Verification items for this drawing (mm, ordinates from the low corner). Give positions to 0.01 mm unless a question says otherwise; leave off trailing zeros. Loops run counter-clockwise (first coordinate to the right, second up) from the corner with the lowest first, then second, coordinate; pieces in that order, holes last. Notation, with made-up numbers: M -6,27.5 L 49,27.5 A21 cw 49,66.5 Z; hole C -31.75,12 d6. An arc over 180 degrees is marked long. Use a Markdown table: item, result.
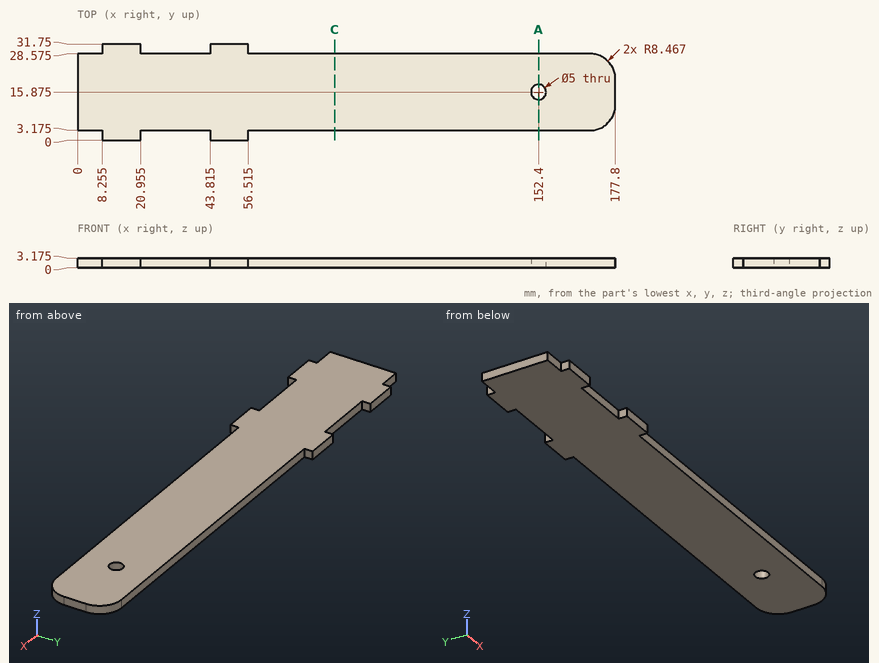
(1) Gauge pin test, flat ends, axial feed: P1, Ø1.6, axis at y = 30, z = 1, coming from the -X side (3 decimals); P2, Ø1, axis at x = 2.5, z = 2, coming from the -Y side (3 decimals); P3, Ø1.6, axis at x = 36.5, z = 1.5, coming from the +Y side (3 decimals). Record the tip position at first contact, or that the pin passes through.
Results below:
| item | result |
|---|---|
| P1 | x = 8.255 |
| P2 | y = 3.175 |
| P3 | y = 28.575 |
(2) Cross-section at C-C on x = 85. Record the cut outline in (y, z) (1 decimal).
Results below:
| item | result |
|---|---|
| outline | M 3.2,0 L 28.6,0 L 28.6,3.2 L 3.2,3.2 Z |
(3) Material ranges on line 1 (X direction, y = 16, z = 2.2); line 2 (Y direction, x = 152.4, z = 1.3) (1 decimal); line 3 (X direction, y = 2, z = 2.35) (1 decimal), recorded low to high.
Results below:
| item | result |
|---|---|
| line 1 | 0 to 149.9, 154.9 to 177.8 |
| line 2 | 3.2 to 13.4, 18.4 to 28.6 |
| line 3 | 8.3 to 21, 43.8 to 56.5 |
(4) Cross-section at A-A on x = 152.4. Record the cut outline in (y, z) (1 decimal).
Results below:
| item | result |
|---|---|
| outline | M 3.2,0 L 13.4,0 L 13.4,3.2 L 3.2,3.2 Z; M 18.4,0 L 28.6,0 L 28.6,3.2 L 18.4,3.2 Z |
